Job drawing, mm, ordinate dimensions from the low corner. One solid piece. A direction names the side the tool comes from. Round coordinates to 2 decimals unless told otherwise and drop trailing zeros. Write each loop counter-clockwise with the first axis right and the second up, starting at its lowest first coordinate (ties: lowest second). Pieces come first, ordered by that corner, then holes. Notation, with made-up numbers: (76.25, 39.5) - (113.25, 39.5) arc R16 cw to (113.25, 53.5) - close; hole circle Ø3 at (-23, -33). An arc over 180 degrees is marked (long way). Write each question's results on one line, items separated by ' | '.
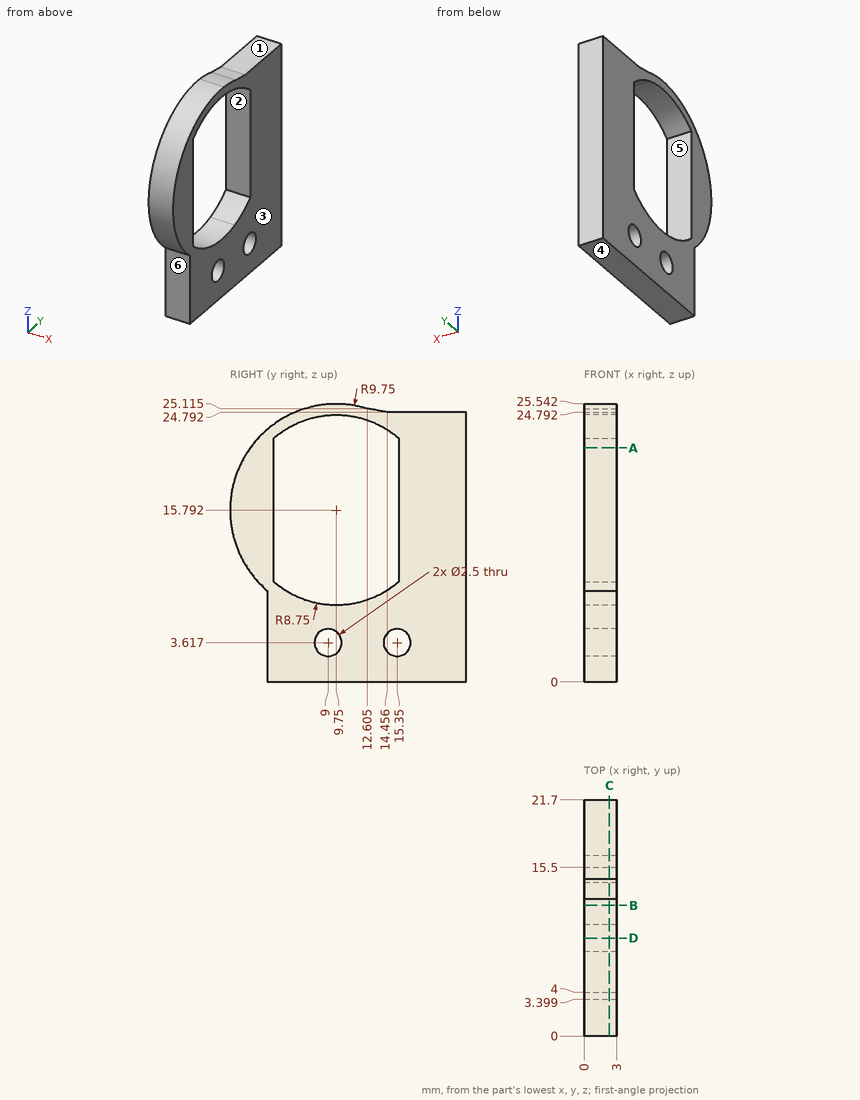
(1) Slice it at C-C, the plane x = 2.3. State how many separate pieces and enclosed holes the cut face has, and give its area (3 significant figures).
Worked answers:
separate pieces: 1 | enclosed holes: 3 | area: 295 mm2
(2) Flat gauge pins, fed straight in: pin 1 Ø0.9 at (x, y) = (1, 18) entering from +Z; pin 2 Ø1.5 at (x, y) = (2.5, 3) entering from +Z; pin 3 Ø1 at (x, y) = (2.5, 9.5) entering from +Z; pin 4 Ø2 at (y, z) = (9, 3.62) entering from +X. Where does each tip first touch, or does it go through?
Worked answers:
pin 1: stops at z = 24.79 | pin 2: stops at z = 23.48 | pin 3: stops at z = 25.54 | pin 4: passes through
(3) Slice it at A-A, the plane z = 21.5. Write the cut outline in (x, y) (1 decimal).
Worked answers:
outline: (0, 1.8) - (3, 1.8) - (3, 4) - (0, 4) - close; (0, 15.5) - (3, 15.5) - (3, 21.7) - (0, 21.7) - close
(4) Two-plate mould, pull along Y, no slides. Class the marked faces 4, 5 and 6: released by +Y, released by -Y, zero draft, split by the parting line, or undercut.
Worked answers:
face 4: zero draft | face 5: undercut | face 6: released by -Y
(5) Drill centre lines: probe 1 along Z at (x, y) = (2.25, 15.35) (1 decimal); probe 2 along Z at (x, y) = (1.35, 9) (1 decimal); probe 3 along Y at (x, z) = (1.1, 2.5) (1 decimal). Where is each one in solid material? Low to high. Write a range as [from, to].
Worked answers:
probe 1: z = [0, 2.4], [4.9, 9.1], [22.5, 24.8] | probe 2: z = [0, 2.4], [4.9, 7.1], [24.5, 25.5] | probe 3: y = [3.4, 8.4], [9.6, 14.8], [15.9, 21.7]
(6) Slice it at D-D, the plane y = 9. Write the cut outline in (x, z).
Worked answers:
outline: (0, 0) - (3, 0) - (3, 2.37) - (0, 2.37) - close; (0, 4.87) - (3, 4.87) - (3, 7.07) - (0, 7.07) - close; (0, 24.51) - (3, 24.51) - (3, 25.51) - (0, 25.51) - close
(7) Tool access for the marked faces 1, 2 and 3: list every direction of +Z, -Z, +X, -X, +Y, -Y with a clear straight run to the whole face (end or side of a thin tool).
Worked answers:
face 1: +Z, +X, -X, +Y | face 2: +X, -X | face 3: +Z, -Z, +X, +Y, -Y
(8) Slice it at B-B, the plane y = 12. Write the cut outline in (x, z).
Worked answers:
outline: (0, 0) - (3, 0) - (3, 7.34) - (0, 7.34) - close; (0, 24.25) - (3, 24.25) - (3, 25.28) - (0, 25.28) - close
